from build123d import *

# Parameters (mm, degrees)
BOSS_EXTRUDE1_DEPTH = 20
FILLET1_R           = 4
SKETCH2_R           = 2.75
CUT_EXTRUDE1_DEPTH  = 1.5
LPATTERN1_COUNT     = 2
LPATTERN1_PITCH     = 30


with BuildPart() as part:
    # Sketch1 → Boss-Extrude1 (new body)
    with BuildSketch(Plane(origin=(0, 0, 0), x_dir=(1, 0, 0), z_dir=(0, 1, 0))):
        with BuildLine():
            Line((-15, -5), (10, -5))
            Line((10, -5), (10, -15))
            ThreePointArc((10, -15), (15, -20), (20, -15))
            Line((20, -15), (20, 0))
            ThreePointArc((20, 0), (18.535533906, 3.535533906), (15, 5))
            Line((15, 5), (-15, 5))
            ThreePointArc((-15, 5), (-20, 0), (-15, -5))
        make_face()
    extrude(amount=BOSS_EXTRUDE1_DEPTH)

    # Fillet1
    fillet1_edges = [part.edges().sort_by_distance(p)[0] for p in [
        (15, 20, 20),
        (20, 20, 7.5),
        (18.535533906, 20, -3.535533906),
        (0, 20, -5),
        (-20, 20, 0),
        (-2.5, 20, 5),
        (10, 20, 10),
    ]]
    fillet(fillet1_edges, radius=FILLET1_R)

    # Sketch2 → Cut-Extrude1 (cut)
    with BuildSketch(Plane.XZ):
        with Locations(Location((-15, 0, 0), (0, 0, 270))):
            Circle(SKETCH2_R)
    cut_extrude1 = extrude(amount=-CUT_EXTRUDE1_DEPTH, mode=Mode.SUBTRACT)

    # LPattern1: Cut-Extrude1 ×2
    with Locations(*[(i * LPATTERN1_PITCH, 0, 0) for i in range(1, LPATTERN1_COUNT)]):
        add(cut_extrude1, mode=Mode.SUBTRACT)


solid = part.part
Part model, mm, in its own coordinate system. A direction names the side the tool comes from. Give positions to 0.01 mm unless a question says otherwise; leave off trailing zeros. Write each loop counter-clockwise with the first axis right and the second up, starting at its lowest first coordinate (ties: lowest second). Pieces come first, ordered by that corner, then holes.
1) Which spindle directions (+Z, -Z, +X, -X, +Y, -Y) get a long thin tool onto all of the face, cutting with end or side? Do faces 4 (the face through (-3, 8, 5)), 5 (the face through (-20, 8, 0)), 6 (the face through (15, 1.5, 0)). Say none if no direction does.
Resolved:
face 4: +Z, -X, +Y, -Y
face 5: -X, +Y, -Y
face 6: -Y
2) Two-plate mould, pull along Z, no slides. Class faces 1 (the face through (11.141, 18.797, 9.654)), 2 (the face through (-15, 1.5, 0)), 3 (the face through (-0.297, 18.797, 3.859)): released by +Z, released by -Z, zero draft, split by the parting line, or undercut.
Resolved:
face 1: zero draft
face 2: undercut
face 3: released by +Z
3) Pin check, flat tips, straight feed: pin 1 (12 mm diameter, centred on x = -4, z = 8, fed in from +Y); pin 2 (3.5 mm diameter, centred on x = -15, z = 0, fed in from -Y); pin 3 (3 mm diameter, centred on x = -15.5, z = -1.5, fed in from -Y); pin 4 (1 mm diameter, centred on y = 7, z = 15.5, fed in from -X). Stop position of each tip, or through.
Resolved:
pin 1: stops at y = 19.87
pin 2: stops at y = 1.5
pin 3: stops at y = 0
pin 4: stops at x = 10
4) Cut at C-C on x = -8. Write the cut outline in (y, z).
Resolved:
outline: (0, -5) - (16, -5) arc R4 ccw to (20, -1) - (20, 1) arc R4 ccw to (16, 5) - (0, 5) - close
5) Cut at A-A on y = 5. Write the cut outline in (x, z).
Resolved:
outline: (-15, -5) - (15, -5) arc R5 ccw to (20, 0) - (20, 15) arc R5 ccw to (10, 15) - (10, 5) - (-15, 5) arc R5 ccw to start
6) Cut at B-B on z = 14.5. Write the cut outline in (x, y), then the cut area to 3 significant figures.
Resolved:
outline: (10, 0) - (20, 0) - (20, 16) arc R4 ccw to (16, 20) - (14, 20) arc R4 ccw to (10, 16) - close
area: 193 mm2
7) Probe L1, parallel to X at y = 0.45, z = 0; L2, parallel to X at y = 14, z = 13; L3, parallel to Y at x = 13, z = -0.5. List the from-to ranges inside material, lowest first.
Resolved:
L1: x = -20 to -17.75, -12.25 to 12.25, 17.75 to 20
L2: x = 10 to 20
L3: y = 1.5 to 20
